```python
from build123d import *

# Parameters (mm, degrees)
SMUSSO1_SIZE = 0.5
SMUSSO2_SIZE = 0.5
SMUSSO3_SIZE = 1
RACCORDO1_R  = 0.5


with BuildPart() as part:
    # Schizzo1 → Rivoluzione1 (revolve)
    with BuildSketch(Plane.XY, mode=Mode.PRIVATE) as rivoluzione1_sk:
        Polygon((0, 0), (0, 10), (3, 10), (3, 6), (32.95, 6), (32.95, 4), (34, 4), (34, 6), (35, 6), (35, 0), align=None)
    revolve(rivoluzione1_sk.sketch.rotate(Axis((-16.326077986, 0, 0), (1, 0, 0)), 90), axis=Axis((-16.326077986, 0, 0), (1, 0, 0)))

    # Smusso1
    smusso1_edges = [part.edges().sort_by_distance(p)[0] for p in [
        (3, 0, -10),
    ]]
    chamfer(smusso1_edges, length=SMUSSO1_SIZE)

    # Smusso2
    smusso2_edges = [part.edges().sort_by_distance(p)[0] for p in [
        (3, 0, -6),
    ]]
    chamfer(smusso2_edges, length=SMUSSO2_SIZE)

    # Smusso3
    smusso3_edges = [part.edges().sort_by_distance(p)[0] for p in [
        (35, 0, -6),
    ]]
    chamfer(smusso3_edges, length=SMUSSO3_SIZE - 0.0001)  # a hair under: the kernel refuses the full size

    # Raccordo1
    raccordo1_edges = [part.edges().sort_by_distance(p)[0] for p in [
        (0, 0, -10),
    ]]
    fillet(raccordo1_edges, radius=RACCORDO1_R)


solid = part.part
```
Check sheet for the modelled part. Datum: model origin and axes. Units: mm. A direction names the side the tool comes from. Give positions to 0.01 mm unless a question says otherwise; leave off trailing zeros. Order: outer loops, then holes, each group sorted by start corner. A loop starts at its lowest first (then second) coordinate and runs counter-clockwise, first axis right, second up. Notation, with made-up numbers: (27.25, 1.25) -> (42.25, 1.25) arc R29 cw to (42.25, 32.25) -> close; hole circle Ø6 at (23.25, 69). An arc over 180 degrees is marked (long way). Return JSON: item names as keys, results as strings.
1. Go/stop test with flat-tipped pins: P1, Ø12, axis at x = 7, y = -5, coming from the -Z side; P2, Ø8, axis at x = 18, y = -7, coming from the -Z side; P3, Ø9.5, axis at y = -1.5, z = 1.5, coming from the -X side; P4, Ø2, axis at x = 27.5, z = -6, coming from the -Y side. Record where each tip stops, or that it passes through.
From the geometry:
{"P1": "z = -9.95", "P2": "z = -5.2", "P3": "x = 0", "P4": "y = -3.32"}
2. Set-up check for faces 1 (the flat face through (0, 0, 0)), 2 (the flat face through (32.95, 3.92, -1.42)), 3 (the flat face through (3, 6, 4)): record each of +Z, -Z, +X, -X, +Y, -Y from which the full face is reachable in a straight line by a thin tool's end or side.
From the geometry:
{"face 1": "+Z, -Z, -X, +Y, -Y", "face 2": "none", "face 3": "+X"}
3. Cross-section at C-C, the plane x = 31.5. Record the cut outline in (y, z).
From the geometry:
{"outline": "circle Ø12 at (0, 0)"}
4. Material ranges on probe 1 along X at (y, z) = (4, 1.5); probe 2 along X at (y, z) = (-7, 3.5); probe 3 along Z at (x, y) = (33, -1), recorded low to high. Write a range as [from, to].
From the geometry:
{"probe 1": "[0, 32.95], [34, 35]", "probe 2": "[0, 3]", "probe 3": "[-3.87, 3.87]"}
5. Mould release check, pull along X, two halves, no side actions. Record for faces 4 (the cylindrical face through (33.482, 3.905, -0.867)), 5 (the flat face through (35, 0, 0)), 6 (the cylindrical face through (18.431, -1.802, 5.723)): +X half, -X half, draft (parallel to the pull), parting line (faces both ways), or undercut.
From the geometry:
{"face 4": "undercut", "face 5": "+X half", "face 6": "draft"}
